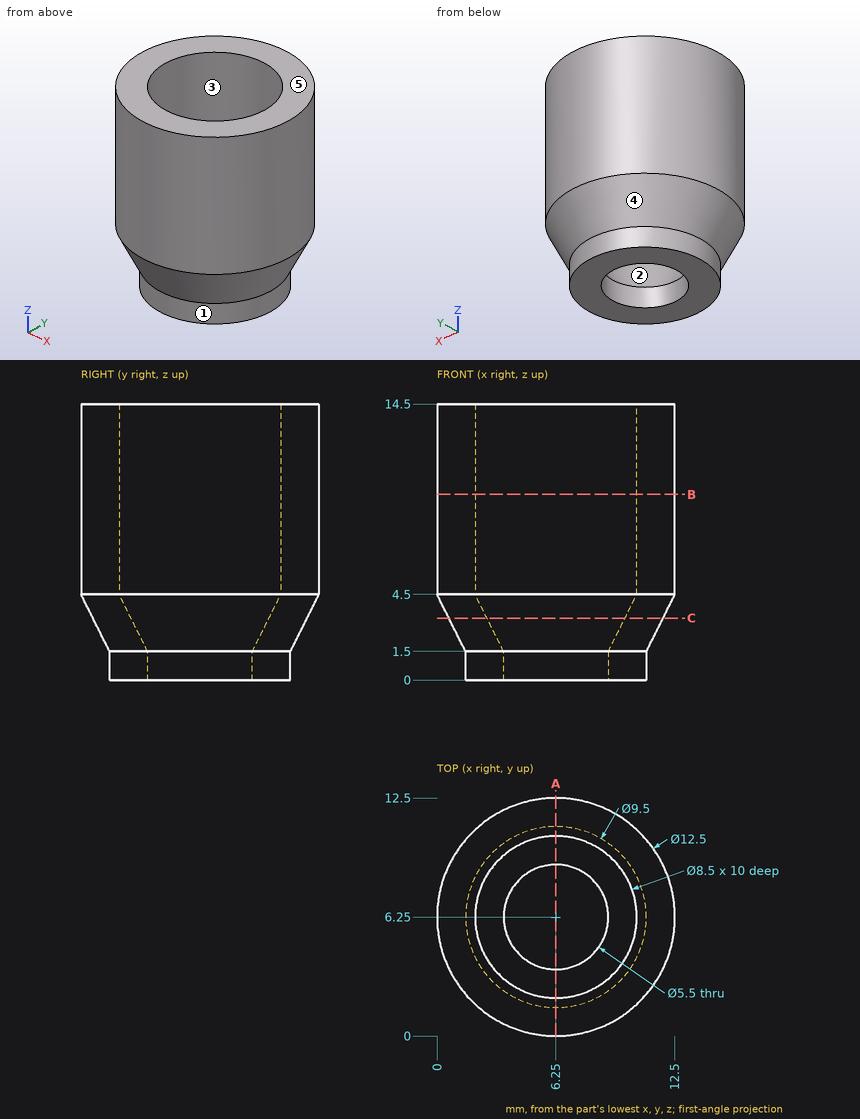
The drawing under review shows one solid part. Ordinate dimensions are in mm from its lowest x, y, z. A direction names the side the tool comes from. Round coordinates to 2 decimals unless told otherwise and drop trailing zeros. Write each loop counter-clockwise with the first axis right and the second up, starting at its lowest first coordinate (ties: lowest second). Pieces come first, ordered by that corner, then holes. Notation, with made-up numbers: (86.5, 0.25) -> (140.5, 0.25) arc R25 ccw to (140.5, 18.25) -> close; hole circle Ø5 at (63, 32.25). An arc over 180 degrees is marked (long way). One line per question, with ' | ' between items. Start each with the question number.
(1) Add section B-B, the plane z = 9.75. Write out the cut boundary in (x, y), plus the area to 3 significant figures.
(2) Add section C-C, the plane z = 3.25. Write out the cut boundary in (x, y) (3 decimals).
(3) Insertion check: P1, Ø1.5, axis at x = 4.5, z = 4.5, coming from the -Y side; P2, Ø6, axis at y = 3, z = 6.5, coming from the -X side (3 decimals); P3, Ø3, axis at x = 10.5, z = 2, coming from the -Y side; P4, Ø5, axis at x = 6.25, y = 6.25, coming from the -Z side. Each pin has a flat end and moves straight along its axis. Give the tip position at first contact, or say it passes through.
(4) Tool access review of the marked faces 1 and 2: name each direction out of +Z, -Z, +X, -X, +Y, -Y from which nothing blocks a thin tool from reaching the whole face with its end or side.
(5) Add section A-A, the plane x = 6.25. Write out the cut boundary in (y, z).
(6) For line 1 along Y through (x, z) = (6.25, 0.9); line 2 along Y through (x, z) = (6.25, 12); line 3 along X through (y, z) = (4, 3.5), list the stretches that pass through material, from the lowest coordinate up. Write a range as from..to.
(7) Mouldability with a two-part tool opening along X and no side actions: class the marked faces 3, 4 and 5 as released by +X, released by -X, zero draft, split by the parting line, or undercut.
Answer list:
1) outline: circle Ø12.5 at (6.25, 6.25); hole circle Ø8.5 at (6.25, 6.25) | area: 66.0 mm²
2) outline: circle Ø11.25 at (6.25, 6.25); hole circle Ø7.25 at (6.25, 6.25)
3) P1: y = 0.08 | P2: x = 0.005 | P3: y = 1.73 | P4: through
4) face 1: -Z | face 2: +Z
5) outline: (0, 4.5) -> (1.5, 1.5) -> (1.5, 0) -> (3.5, 0) -> (3.5, 1.5) -> (2, 4.5) -> (2, 14.5) -> (0, 14.5) -> close; (9, 0) -> (11, 0) -> (11, 1.5) -> (12.5, 4.5) -> (12.5, 14.5) -> (10.5, 14.5) -> (10.5, 4.5) -> (9, 1.5) -> close
6) line 1: 1.5..3.5, 9..11 | line 2: 0..2, 10.5..12.5 | line 3: 0.96..3.25, 9.25..11.54
7) face 3: undercut | face 4: split by the parting line | face 5: zero draft
